Can you work these out from the drawing? Everything is in mm from the part's minimum corner. A direction names the side the tool comes from. Round coordinates to 2 decimals unless told otherwise and drop trailing zeros. Write each loop counter-clockwise with the first axis right and the second up, starting at its lowest first coordinate (ties: lowest second). Pieces come first, ordered by that corner, then holes.
Q1. If we section it at C-C (z = 25): Please give me the cut outline in (x, y), plus the area to 3 significant figures.
Q2. If we section it at A-A (y = 5.25): Please give me the cut outline in (x, z).
Q3. I'm going to push flat-ended pins straight in: pin 1 Ø4 at (x, z) = (84.5, 28.5) entering from +Y; pin 2 Ø6 at (x, z) = (68, 23) entering from -Y. Where does each tip first touch, or does it pass through?
Q4. For the marked faces 1 and 2, which set-ups out of +Z, -Z, +X, -X, +Y, -Y let a thin tool reach every point of the face, with its end or its side?
Q5. Please list where these lines run through material, in increasing order: line 1 along X through (y, z) = (11.75, 6); line 2 along Z through (x, y) = (81, 3.25); line 3 along Y through (x, z) = (44, 23).
Q6. We'd pull the mould along Z, two halves only. Please class the marked faces 3, 4 and 5: +Z half, -Z half, draft (parallel to the pull), parting line (faces both ways), or undercut.
Q7. If we section it at B-B (x = 23): Please give me the cut outline in (y, z).
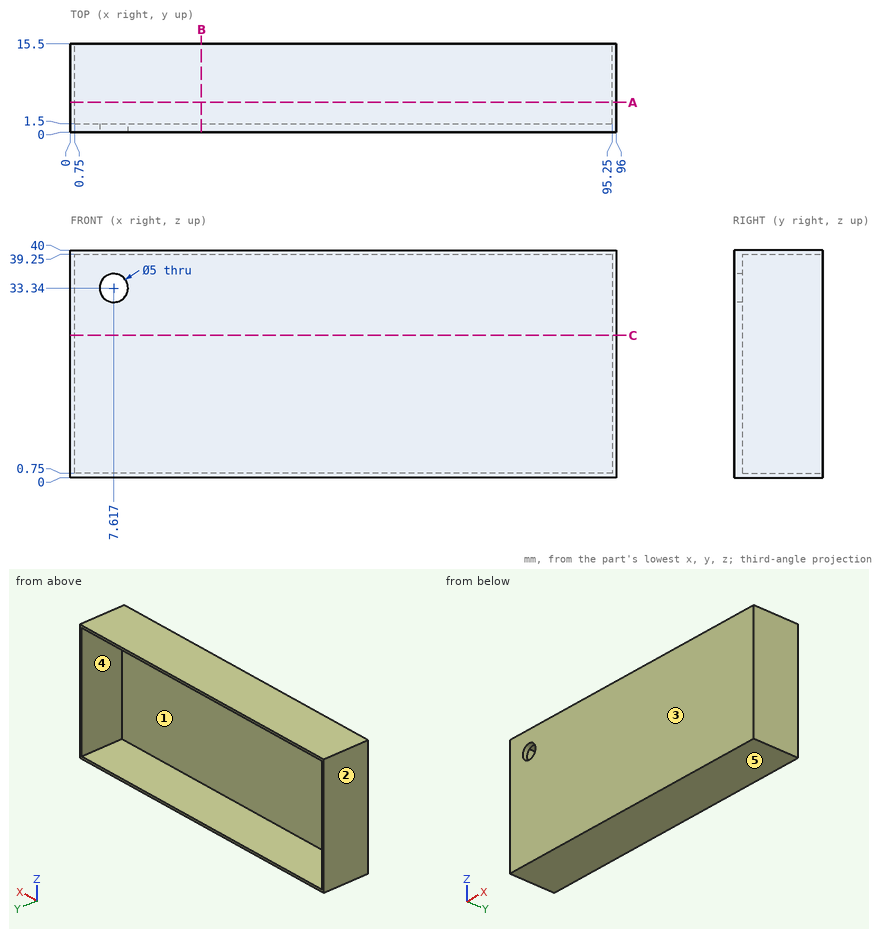
A:
1. outline: (0, 0) - (96, 0) - (96, 15.5) - (95.25, 15.5) - (95.25, 1.5) - (0.75, 1.5) - (0.75, 15.5) - (0, 15.5) - close
1. area: 165 mm2
2. outline: (0, 0) - (96, 0) - (96, 40) - (0, 40) - close; hole (0.75, 0.75) - (95.25, 0.75) - (95.25, 39.25) - (0.75, 39.25) - close
3. pin 1: stops at y = 1.5
3. pin 2: stops at y = 0
4. face 1: +Y
4. face 2: +Z, -Z, -X, +Y, -Y
5. line 1: x = 0 to 0.75, 95.25 to 96
5. line 2: z = 0 to 0.75, 39.25 to 40
5. line 3: y = 0 to 1.5
6. face 3: draft
6. face 4: undercut
6. face 5: -Z half
7. outline: (0, 0) - (15.5, 0) - (15.5, 0.75) - (1.5, 0.75) - (1.5, 39.25) - (15.5, 39.25) - (15.5, 40) - (0, 40) - close
